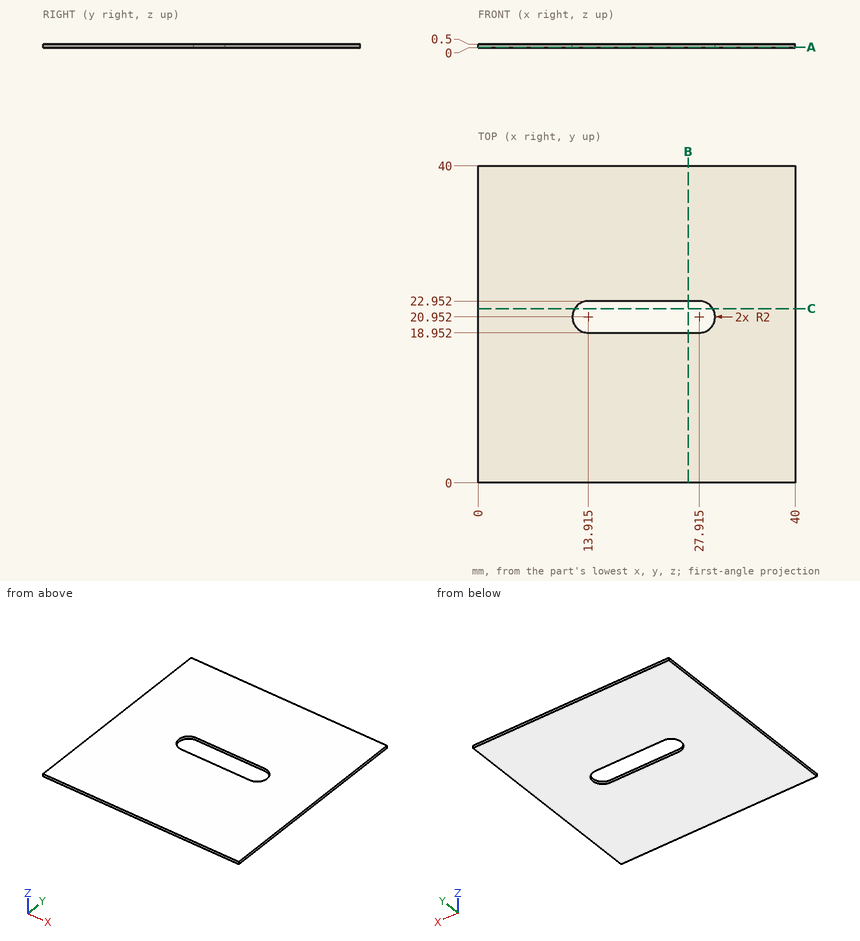
The figure shows three views and two pictorial views of one solid part (mm, origin at its lowest corner). Answer the questions. Coordinates: 2 decimals unless noted, no trailing zeros. Write each loop counter-clockwise with the first axis right and the second up, starting at its lowest first coordinate (ties: lowest second). Pieces come first, ordered by that corner, then holes. Notation, with made-up numbers: (57.5, 73.25) -> (93.5, 73.25) arc R15 ccw to (93.5, 89.25) -> close; hole circle Ø7 at (-24, -34). An arc over 180 degrees is marked (long way). Return JSON: item names as keys, results as strings.
1. A cutting plane is placed at A-A (z = 0.1). Determine the outline of the cut face in (x, y) (1 decimal), and give its area (3 significant figures).
Found:
{"outline": "(0, 0) -> (40, 0) -> (40, 40) -> (0, 40) -> close; hole (13.9, 19) -> (27.9, 19) arc R2 ccw to (27.9, 23) -> (13.9, 23) arc R2 ccw to start", "area": "1,530 mm2"}
2. A cutting plane is placed at B-B (x = 26.5). Determine the outline of the cut face in (y, z).
Found:
{"outline": "(0, 0) -> (18.95, 0) -> (18.95, 0.5) -> (0, 0.5) -> close; (22.95, 0) -> (40, 0) -> (40, 0.5) -> (22.95, 0.5) -> close"}
3. Find the intervals of material crossed by line 1 along Y through (x, z) = (18, 0.15), in increasing order. Write a range as from..to.
Found:
{"line 1": "0..18.95, 22.95..40"}
4. A cutting plane is placed at C-C (y = 22). Determine the outline of the cut face in (x, z).
Found:
{"outline": "(0, 0) -> (12.21, 0) -> (12.21, 0.5) -> (0, 0.5) -> close; (29.62, 0) -> (40, 0) -> (40, 0.5) -> (29.62, 0.5) -> close"}
